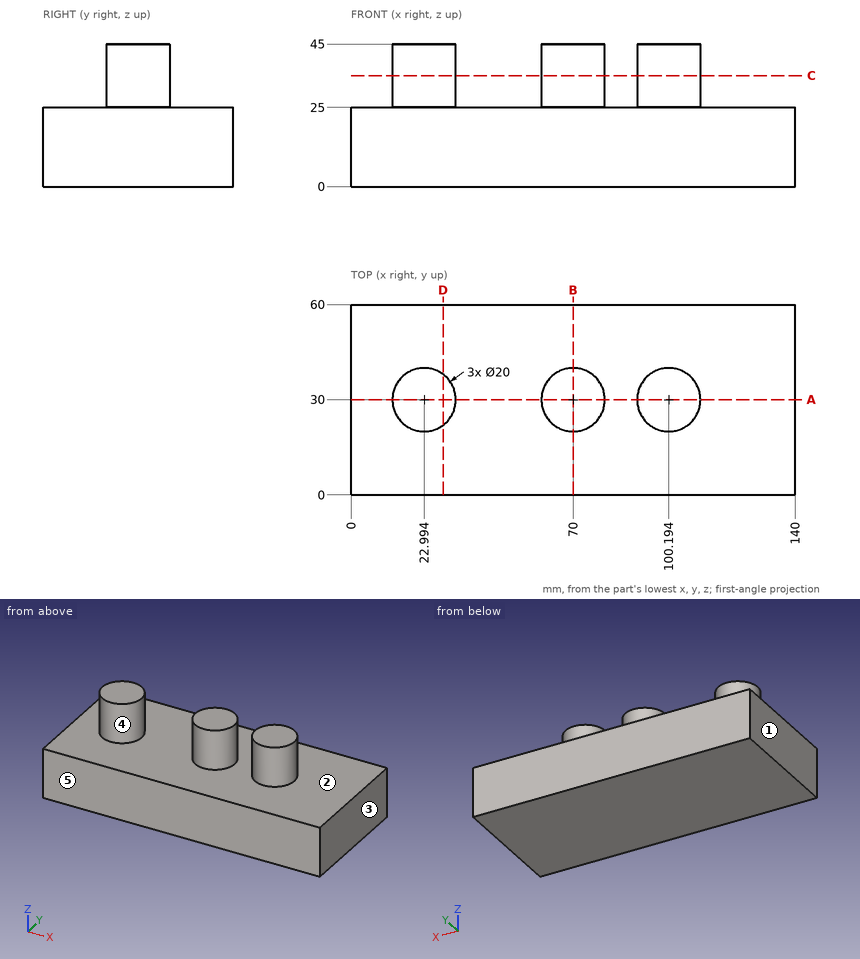
The figure shows three views and two pictorial views of one solid part (mm, origin at its lowest corner). Answer the questions. A direction names the side the tool comes from. Coordinates: 2 decimals unless noted, no trailing zeros. Loops run counter-clockwise (first coordinate to the right, second up) from the corner with the lowest first, then second, coordinate; pieces in that order, holes last.
1) Flat-ended cylindrical pins translate along their axes: pin 1 Ø12 at (x, y) = (30.5, 53) entering from -Z; pin 2 Ø10 at (x, z) = (23.5, 32) entering from -Y. Find the tip coordinate at first contact, or state that the pin passes through.
2) A tool of negligible diameter and unlimited length cuts with its end or side. For the marked faces 1 and 2, from which of +Z, -Z, +X, -X, +Y, -Y can it reach the whole face along a straight path? Write none if from no direction.
3) Find section C-C on z = 35. Write down the section's boundary in (x, y) (1 decimal).
4) Find section B-B on x = 70. Write down the section's boundary in (y, z).
5) Find the intervals of material crossed by L1, parallel to Z at x = 20.5, y = 17; L2, parallel to X at y = 33, z = 32 (1 decimal); L3, parallel to Y at x = 71.5, z = 35, in increasing order.
6) Determine the mould class of the marked faces 3, 4 and 5 for opening direction X: pulls with the +X half, pulls with the -X half, needs draft (parallel to the pull), parting line crosses it, or undercut.
7) Find section A-A on y = 30. Write down the section's boundary in (x, z) (1 decimal), then the cut area to 3 significant figures.
8) Find section D-D on x = 29. Write down the section's boundary in (y, z) (1 decimal), then the cut area to 3 significant figures.
Values:
1. pin 1: stops at z = 0
1. pin 2: stops at y = 20
2. face 1: +Z, -Z, -X, +Y, -Y
2. face 2: +Z
3. outline: circle Ø20 at (23, 30); circle Ø20 at (70, 30); circle Ø20 at (100.2, 30)
4. outline: (0, 0) - (60, 0) - (60, 25) - (40, 25) - (40, 45) - (20, 45) - (20, 25) - (0, 25) - close
5. L1: z = 0 to 25
5. L2: x = 13.5 to 32.5, 60.5 to 79.5, 90.7 to 109.7
5. L3: y = 20.11 to 39.89
6. face 3: pulls with the +X half
6. face 4: undercut
6. face 5: needs draft
7. outline: (0, 0) - (140, 0) - (140, 25) - (110.2, 25) - (110.2, 45) - (90.2, 45) - (90.2, 25) - (80, 25) - (80, 45) - (60, 45) - (60, 25) - (33, 25) - (33, 45) - (13, 45) - (13, 25) - (0, 25) - close
7. area: 4,700 mm2
8. outline: (0, 0) - (60, 0) - (60, 25) - (38, 25) - (38, 45) - (22, 45) - (22, 25) - (0, 25) - close
8. area: 1,820 mm2
